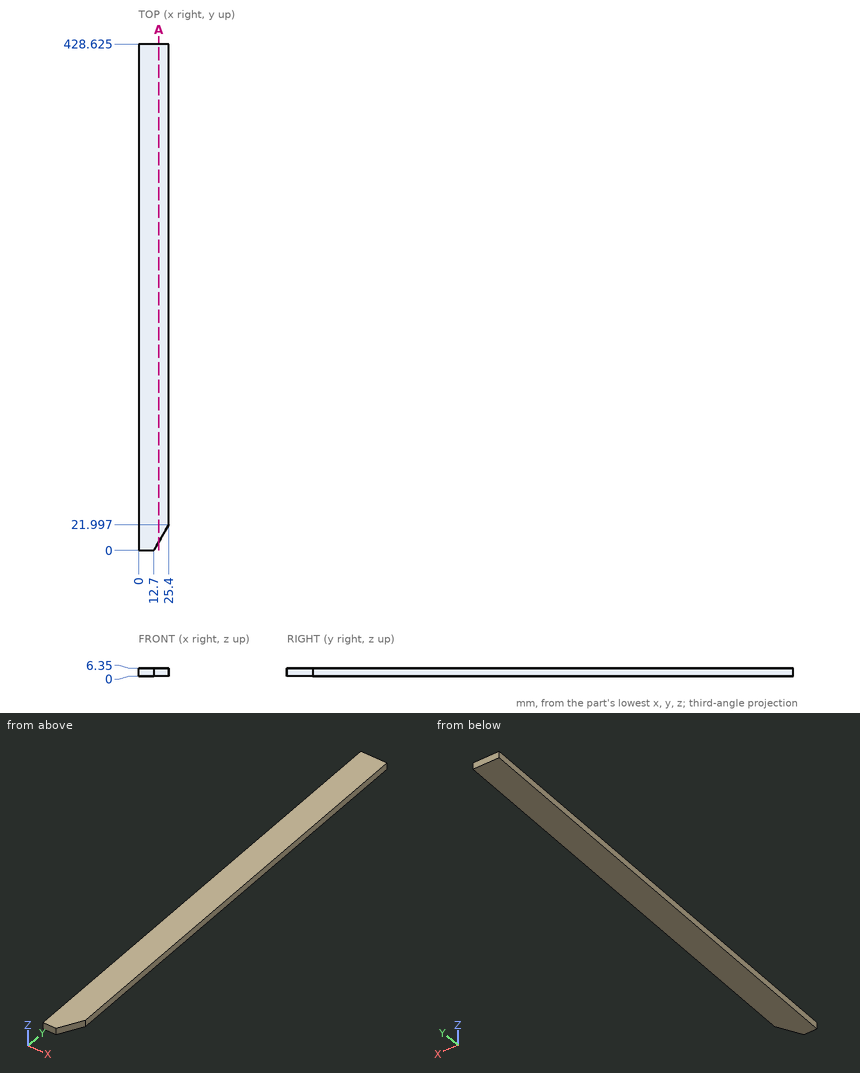
Design review of the part shown in the three views and the two pictorial views. Dimensions are in mm from the part's minimum x, y and z. Coordinates: 2 decimals unless noted, no trailing zeros. Order: outer loops, then holes, each group sorted by start corner. A loop starts at its lowest first (then second) coordinate and runs counter-clockwise, first axis right, second up.
Item 1: For pin 1 Ø3 at (x, z) = (16.5, 2) entering from -Y, flat-tipped, find the tip position at first contact; note if it passes through.
Item 2: For line 1 (Y direction, x = 12.75, z = 0.5) (3 decimals); line 2 (Y direction, x = 17, z = 0.5) (3 decimals); line 3 (X direction, y = 21.5, z = 3.5), list the stretches that pass through material, from the lowest coordinate up.
Item 3: Take a section at A-A, the plane x = 17. Write out the cut boundary in (y, z) (3 decimals), then the cut area to 3 significant figures.
The answers:
1. pin 1: stops at y = 3.98
2. line 1: y = 0.087 to 428.625
2. line 2: y = 7.448 to 428.625
2. line 3: x = 0 to 25.11
3. outline: (7.448, 0) - (428.625, 0) - (428.625, 6.35) - (7.448, 6.35) - close
3. area: 2,670 mm2
